```python
from build123d import *

# Parameters (mm, degrees)
SKETCH_1_R          = 1.175
SKETCH_1_R_2        = 1.35
EXTRUDE_1_DEPTH     = 4
SKETCH_1_5_R        = 1.175
EXTRUDE_2_DEPTH     = 12
SKETCH_1_6_R        = 1.175
CUT_EXTRUDE_1_DEPTH = 8
SKETCH_3_R          = 1.625
CUT_EXTRUDE_2_DEPTH = 1
CHAMFER_1_SIZE      = 10
FILLET_1_R          = 12


with BuildPart() as part:
    # 草图1 → 凸台-拉伸1 (new body)
    with BuildSketch(Plane(origin=(0, 0, 0), x_dir=(0, 0, -1), z_dir=(1, 0, 0))):
        with BuildLine():
            ThreePointArc((-22.696428571, -2.043453335), (0, -11.927768877), (22.696428571, -2.043453335))
            ThreePointArc((22.696428571, -2.043453335), (22.543453335, 2.196428571), (18.303571429, 2.043453335))
            ThreePointArc((18.303571429, 2.043453335), (0, -5.927768877), (-18.303571429, 2.043453335))
            ThreePointArc((-18.303571429, 2.043453335), (-22.543453335, 2.196428571), (-22.696428571, -2.043453335))
        make_face()
        with Locations((20.5, 0)):
            Circle(SKETCH_1_R, mode=Mode.SUBTRACT)
        with Locations((-20.5, 0)):
            Circle(SKETCH_1_R_2, mode=Mode.SUBTRACT)
    extrude(amount=EXTRUDE_1_DEPTH)

    # 草图1<5> → 凸台-拉伸2 (add)
    # profile 1 of 2: a face of its own
    with BuildSketch(Plane(origin=(0, 0, 0), x_dir=(0, 0, -1), z_dir=(1, 0, 0))):
        with BuildLine():
            Line((-5.226102274, -5.375424287), (-6.48036682, -11.242861585))
            ThreePointArc((-6.48036682, -11.242861585), (4.046311959, -11.66255958), (14.105677022, -8.532657498))
            Line((14.105677022, -8.532657498), (11.375545986, -3.189775829))
            ThreePointArc((11.375545986, -3.189775829), (3.263154806, -5.713890412), (-5.226102274, -5.375424287))
        make_face()
    # profile 2 of 2: a face of its own
    with BuildSketch(Plane(origin=(0, 0, 0), x_dir=(0, 0, -1), z_dir=(1, 0, 0))):
        with BuildLine():
            Line((11.375545986, -3.189775829), (14.105677022, -8.532657498))
            ThreePointArc((14.105677022, -8.532657498), (18.684918697, -5.663852102), (22.696428571, -2.043453335))
            ThreePointArc((22.696428571, -2.043453335), (22.543453335, 2.196428571), (18.303571429, 2.043453335))
            ThreePointArc((18.303571429, 2.043453335), (15.06848282, -0.876223091), (11.375545986, -3.189775829))
        make_face()
        with Locations((20.5, 0)):
            Circle(SKETCH_1_5_R, mode=Mode.SUBTRACT)
    extrude(amount=EXTRUDE_2_DEPTH)

    # 草图1<6> → 切除-拉伸1 (cut)
    with BuildSketch(Plane(origin=(0, 0, 0), x_dir=(0, 0, -1), z_dir=(1, 0, 0))):
        with BuildLine():
            Line((11.375545986, -3.189775829), (14.105677022, -8.532657498))
            ThreePointArc((14.105677022, -8.532657498), (18.684918697, -5.663852102), (22.696428571, -2.043453335))
            ThreePointArc((22.696428571, -2.043453335), (22.543453335, 2.196428571), (18.303571429, 2.043453335))
            ThreePointArc((18.303571429, 2.043453335), (15.06848282, -0.876223091), (11.375545986, -3.189775829))
        make_face()
        with Locations((20.5, 0)):
            Circle(SKETCH_1_6_R, mode=Mode.SUBTRACT)
    extrude(amount=CUT_EXTRUDE_1_DEPTH, mode=Mode.SUBTRACT)

    # 草图3 → 切除-拉伸2 (cut)
    with BuildSketch(Plane.ZY):
        with Locations((20.5, 0)):
            Circle(SKETCH_3_R)
    extrude(amount=-CUT_EXTRUDE_2_DEPTH, mode=Mode.SUBTRACT)

    # 倒角1
    # the kernel refuses this chamfer: 10 mm, written as the material it adds along each edge
    # the kernel refuses this chamfer: 10 mm, written as the material it takes off along each edge
    with BuildSketch(Plane(origin=(12, 19.773223518, -0.149849051), x_dir=(-0.9996219169112968, 0.005747850531589265, 0.02688838866222917), z_dir=(0, -0.9779062163770691, 0.20904409097385418))) as chamfer_1_2_piece_1_section:
        Polygon((CHAMFER_1_SIZE * 0.999621916911, CHAMFER_1_SIZE * 0.0274958766106), (-CHAMFER_1_SIZE * 0.0274958766106, CHAMFER_1_SIZE * 0.999621916911), (0, 0), align=None)
    chamfer_1_2_piece_1 = extrude(amount=57.433659759, mode=Mode.PRIVATE)
    chamfer_1_2_piece_1 = split(chamfer_1_2_piece_1, bisect_by=Plane(origin=(4, -8.720114363, 2.38807711), z_dir=(1, 0, 0)), keep=Keep.TOP, mode=Mode.PRIVATE)
    add(chamfer_1_2_piece_1, mode=Mode.SUBTRACT)
    with BuildSketch(Plane(origin=(0, 19.710553993, 0.32617325), x_dir=(-0.02749587661058638, -0.45484980336482234, 0.8901436025430942), z_dir=(0, -0.8904802780770589, -0.45502183942730046))) as chamfer_1_2_piece_2_section:
        Polygon((CHAMFER_1_SIZE * 0.999621916911, -CHAMFER_1_SIZE * 0.0274958766106), (-CHAMFER_1_SIZE * 0.0274958766106, -CHAMFER_1_SIZE * 0.999621916911), (0, 0), align=None)
    chamfer_1_2_piece_2 = extrude(amount=57.433659759, mode=Mode.PRIVATE)
    chamfer_1_2_piece_2 = split(chamfer_1_2_piece_2, bisect_by=Plane(origin=(8, -7.155033318, -9.499893675), z_dir=(-1, 0, 0)), keep=Keep.TOP, mode=Mode.PRIVATE)
    add(chamfer_1_2_piece_2, mode=Mode.SUBTRACT)

    # 圆角1
    fillet_1_edges = [part.edges().sort_by_distance(p)[0] for p in [
        (12, -8.568786932, -4.317191604),
        (8, -6.706828834, -10.92672743),
        (4, -8.656473826, 3.88229654),
        (0, -8.74431349, -2.983935031),
    ]]
    fillet(fillet_1_edges, radius=FILLET_1_R)


solid = part.part
```
Input: part model. Units: mm. Frame: model coordinates. A direction names the side the tool comes from. Coordinates: 2 decimals unless noted, no trailing zeros. Loops run counter-clockwise (first coordinate to the right, second up) from the corner with the lowest first, then second, coordinate; pieces in that order, holes last. Notation, with made-up numbers: (-16, 67.5) - (-8, 67.5) arc R33 ccw to (-8, 104.5) - close; hole circle Ø10 at (-14.75, 23). An arc over 180 degrees is marked (long way). Answer in a Markdown table with one row per item.
(1) Cut plane D-D on z = -20.5. Output: boundary loops of the cut face in (x, y) (3 decimals), plus the area to 3 significant figures.
Model answer:
| item | result |
|---|---|
| outline | (8, -4.182) - (12, -4.182) - (12, -1.175) - (8, -1.175) - close; (8, 1.175) - (12, 1.175) - (12, 3) - (8, 3) - close |
| area | 19.3 mm² |
(2) Cut plane C-C on x = 9.25. Output: boundary loops of the cut face in (y, z) (3 decimals).
Model answer:
| item | result |
|---|---|
| outline | (-11.916, -0.867) arc R31 ccw to (-2.043, -22.696) arc R3 ccw to (2.043, -18.304) arc R25 cw to (-5.834, -2.168) - close; hole circle Ø2.35 at (0, -20.5) |
(3) Pin query (flat end, axial travel): P1, Ø1, axis at y = 0, z = 20, coming from the -X side; P2, Ø5, axis at y = -3, z = 10, coming from the +X side; P3, Ø4, axis at x = 7, z = -6.5, coming from the +Y side; P4, Ø6, axis at x = 1.5, z = 11, coming from the +Y side. Return the tip coordinate at first contact, or that it passes through.
Model answer:
| item | result |
|---|---|
| P1 | passes through |
| P2 | stops at x = 4 |
| P3 | stops at y = -4.44 |
| P4 | stops at y = -1.64 |
(4) Material intervals for L1, parallel to X at y = -4, z = -15.5; L2, parallel to Z at x = 3.2, y = 0; L3, parallel to Z at x = 8.5, y = -0.25, sorted ascending. Write a range as from..to.
Model answer:
| item | result |
|---|---|
| L1 | x = 8..12 |
| L2 | z = 16.16..19.15, 21.85..23.5 |
| L3 | z = -23.49..-21.65, -19.35..-15.86 |
(5) Cut plane A-A on y = 0. Output: boundary loops of the cut face in (x, z) (3 decimals), plus the area to 3 significant figures.
Model answer:
| item | result |
|---|---|
| outline | (0, 16.163) - (4, 16.163) - (4, 19.15) - (1, 19.15) - (1, 18.875) - (0, 18.875) - close; (0, 22.125) - (1, 22.125) - (1, 21.85) - (4, 21.85) - (4, 23.5) - (0, 23.5) - close; (8, -23.5) - (12, -23.5) - (12, -21.675) - (8, -21.675) - close; (8, -19.325) - (12, -19.325) - (12, -16.163) - (8, -16.163) - close |
| area | 37.9 mm² |
(6) Set-up query: faces 4 (the face through (0.49, -0.62, 22)), 5 (the face through (2.479, 0.406, 19.212)). Return all of +Z, -Z, +X, -X, +Y, -Y with unobstructed straight access to the full face (end or side cutting, diameter ignored); none if empty.
Model answer:
| item | result |
|---|---|
| face 4 | -X |
| face 5 | +X, -X |
(7) Mould query, pull axis Z, two halves, no side actions, for faces 1 (the face through (5.916, -5.926, -0.288)), 2 (the face through (8, -2, -19)), 3 (the face through (5.916, -11.926, 0.357)). Classes: pulls with the +Z half, pulls with the -Z half, needs draft (parallel to the pull), parting line crosses it, or undercut.
Model answer:
| item | result |
|---|---|
| face 1 | undercut |
| face 2 | needs draft |
| face 3 | parting line crosses it |
(8) Cut plane B-B on z = 20.5. Output: boundary loops of the cut face in (x, y) (3 decimals).
Model answer:
| item | result |
|---|---|
| outline | (0, -4.182) - (4, -4.182) - (4, -1.35) - (1, -1.35) - (1, -1.625) - (0, -1.625) - close; (0, 1.625) - (1, 1.625) - (1, 1.35) - (4, 1.35) - (4, 3) - (0, 3) - close |
